Build history of the part. All positions in model axes, mm. A direction names the side the tool comes from. Round coordinates to 2 decimals unless told otherwise and drop trailing zeros. Write each loop counter-clockwise with the first axis right and the second up, starting at its lowest first coordinate (ties: lowest second). Pieces come first, ordered by that corner, then holes.
from build123d import *

# Parameters (mm, degrees)
SKETCH1_R               = 4.025
SKETCH1_R_2             = 2.125
BOSS_EXTRUDE1_DEPTH     = 5
SKETCH2_W               = 28.904595792
SKETCH2_H               = 55.332112
CUT_EXTRUDE1_DEPTH      = 1
CUT_EXTRUDE1_DEPTH_BACK = 6
SKETCH3_W               = 24.207106467
SKETCH3_H               = 21.100530829
CUT_EXTRUDE2_DEPTH      = 1
CUT_EXTRUDE2_DEPTH_BACK = 6
FILLET1_R               = 4
BOSS_EXTRUDE2_DEPTH     = 5
CUT_EXTRUDE3_DEPTH      = 6
CIRPATTERN1_COUNT       = 3
CIRPATTERN1_ANGLE       = 120


with BuildPart() as part:
    # Sketch1 → Boss-Extrude1 (new body)
    with BuildSketch(Plane(origin=(0, 0, 0), x_dir=(1, 0, 0), z_dir=(0, 1, 0))):
        with BuildLine():
            Line((-47.75734818, 56.526415903), (-38.07680463, 45.068358625))
            ThreePointArc((-38.07680463, 45.068358625), (-56.716415256, 16.255714087), (-56.169167779, -18.056151058))
            Line((-56.169167779, -18.056151058), (-70.449464672, -22.646697938))
            ThreePointArc((-70.449464672, -22.646697938), (-71.135842864, 20.388522754), (-47.75734818, 56.526415903))
        make_face()
        with Locations((-49.366374859, 46.034889304)):
            Circle(SKETCH1_R, mode=Mode.SUBTRACT)
        with Locations((-63, 0)):
            Circle(SKETCH1_R_2, mode=Mode.SUBTRACT)
        with Locations((-63, -15)):
            Circle(SKETCH1_R_2, mode=Mode.SUBTRACT)
        with Locations((-63, 15)):
            Circle(SKETCH1_R_2, mode=Mode.SUBTRACT)
    extrude(amount=BOSS_EXTRUDE1_DEPTH)

    # Sketch2 → Cut-Extrude1 (cut, two sides)
    with BuildSketch(Plane(origin=(0, 5, 0), x_dir=(1, 0, 0), z_dir=(0, 1, 0))) as cut_extrude1_sk:
        with Locations((-84.452297896, 0)):
            Rectangle(SKETCH2_W, SKETCH2_H)
    extrude(amount=CUT_EXTRUDE1_DEPTH, mode=Mode.SUBTRACT)
    extrude(cut_extrude1_sk.sketch, amount=-CUT_EXTRUDE1_DEPTH_BACK, mode=Mode.SUBTRACT)

    # Sketch3 → Cut-Extrude2 (cut, two sides)
    with BuildSketch(Plane(origin=(0, 5, 0), x_dir=(1, 0, 0), z_dir=(0, 1, 0))) as cut_extrude2_sk:
        with Locations((-57.896446767, -14.949043558)):
            Rectangle(SKETCH3_W, SKETCH3_H)
    extrude(amount=CUT_EXTRUDE2_DEPTH, mode=Mode.SUBTRACT)
    extrude(cut_extrude2_sk.sketch, amount=-CUT_EXTRUDE2_DEPTH_BACK, mode=Mode.SUBTRACT)

    # Fillet1
    fillet1_edges = [part.edges().sort_by_distance(p)[0] for p in [
        (-70, 2.5, -24),
        (-58.835794809, 2.5, 4.398778143),
        (-70, 2.5, 4.398778143),
        (-47.75734818, 2.5, -56.526415903),
        (-38.07680463, 2.5, -45.068358625),
    ]]
    fillet(fillet1_edges, radius=FILLET1_R)

    # Sketch4 → Boss-Extrude2 (add)
    with BuildSketch(Plane(origin=(0, 0, 0), x_dir=(1, 0, 0), z_dir=(0, 1, 0))):
        with BuildLine():
            ThreePointArc((-54.349205626, 50.221149408), (34.402166182, 65.517104347), (72.198801996, -16.227538025))
            Line((72.198801996, -16.227538025), (57.563909699, -12.938172209))
            ThreePointArc((57.563909699, -12.938172209), (25.337317552, 53.282458082), (-46.367196347, 36.484011606))
            Line((-46.367196347, 36.484011606), (-43.532667136, 51.526011005))
            Line((-43.532667136, 51.526011005), (-54.349205626, 50.221149408))
        make_face()
    extrude(amount=BOSS_EXTRUDE2_DEPTH)

    # Sketch5 → Cut-Extrude3 (cut, through all)
    with BuildSketch(Plane(origin=(0, 5, 0), x_dir=(1, 0, 0), z_dir=(0, 1, 0))):
        Polygon((-36.295708479, 58.895004423), (-34.448714026, 55.34696109), (-25.578605694, 59.964447223), (-27.425600147, 63.512490555), align=None)
    cut_extrude3 = extrude(amount=-CUT_EXTRUDE3_DEPTH, mode=Mode.SUBTRACT)

    # CirPattern1: Cut-Extrude3 ×3 about axis
    cirpattern1_axis = Axis((0, 0, 0), (0, -1, 0))
    for i in range(1, CIRPATTERN1_COUNT):
        add(cut_extrude3.rotate(cirpattern1_axis, i * CIRPATTERN1_ANGLE / (CIRPATTERN1_COUNT - 1)), mode=Mode.SUBTRACT)


solid = part.part
1) Slice it at B-B (y = 2.7). Count the separate pieces of the cut face and the enclosed holes in it, plus the area to 3 significant figures.
Results:
separate pieces: 1
enclosed holes: 6
area: 3,130 mm2
2) Slice it at C-C (x = -31). Write the cut outline in (y, z).
Results:
outline: (0, -67.19) - (5, -67.19) - (5, -61.65) - (0, -61.65) - close; (0, -57.14) - (5, -57.14) - (5, -50.2) - (0, -50.2) - close
3) Slice it at D-D (z = -15). Write the cut outline in (x, y) (3 decimals), plus the area to 3 significant figures.
Results:
outline: (-70, 0) - (-65.125, 0) - (-65.125, 5) - (-70, 5) - close; (-60.875, 0) - (-57.061, 0) - (-57.061, 5) - (-60.875, 5) - close; (57.061, 0) - (72.464, 0) - (72.464, 5) - (57.061, 5) - close
area: 120 mm2
4) Which spindle directions (+Z, -Z, +X, -X, +Y, -Y) get a long thin tool onto all of the face, cutting with end or side? Do faces 4 (the flat face through (-65, 3, 4.399)), 5 (the flat face through (-35.385, 2.535, -57.146)), 6 (the flat face through (8, 0, -59)). Say none if no direction does.
Results:
face 4: +Z, -X, +Y, -Y
face 5: +Y, -Y
face 6: +Z, -Z, +X, -X, -Y
5) Slice it at A-A (z = -39.5). Write the cut outline in (x, y).
Results:
outline: (-62.58, 0) - (-43.83, 0) - (-43.83, 5) - (-62.58, 5) - close; (43.83, 0) - (62.58, 0) - (62.58, 5) - (43.83, 5) - close
6) Pin check, flat tips, straight feed: pin 1 Ø1.5 at (x, y) = (-64, 1.5) entering from +Z; pin 2 Ø3 at (x, y) = (58, 3.5) entering from -Z. Stop position of each tip, or through.
Results:
pin 1: stops at z = 4.4
pin 2: stops at z = -47.79
7) Wall check: L1, parallel to X at y = 4.05, z = 0 (3 decimals); L2, parallel to X at y = 1.1, z = -47; L3, parallel to X at y = 1.95, z = 1 (3 decimals). Give the ranges that are in metal, low to high.
Results:
L1: x = -70 to -65.125, -60.875 to -59, 59 to 65.062, 69.066 to 74
L2: x = -57.16 to -53.27, -45.46 to -35.67, 35.67 to 57.16
L3: x = -69.955 to -64.875, -61.125 to -59.044, 58.992 to 65.018, 69.022 to 73.993
8) Mould opens along Z. For faces 1 (the flat face through (64.984, 2.465, 14.606)), 2 (the flat face through (-70, 3, -11)), 3 (the flat face through (-26.489, 2.535, -61.714)) say: released by +Z, released by -Z, zero draft, split by the parting line, or undercut.
Results:
face 1: released by +Z
face 2: zero draft
face 3: undercut
